Can you work these out from the model? Positions are in its coordinate system, mm. Face numbers are marked on the shaded views. A direction names the side the tool comes from. Coordinates: 2 decimals unless noted, no trailing zeros. Loops run counter-clockwise (first coordinate to the right, second up) from the corner with the lowest first, then second, coordinate; pieces in that order, holes last. Notation, with made-up numbers: M 31,42.5 L 45,42.5 A12 cw 45,60.5 Z; hole C -20.75,20.5 d4. An arc over 180 degrees is marked long. Return JSON: item names as keys, results as strings. Group by question number.
```python
from build123d import *

# Parameters (mm, degrees)
SKETCH1_W                       = 45
SKETCH1_H                       = 20
SKETCH1_R                       = 2.5
BOSS_EXTRUDE1_DEPTH             = 25
SKETCH9_W                       = 45
SKETCH9_H                       = 45
BOSS_EXTRUDE4_DEPTH             = 15
CUT_EXTRUDE2_START              = -2.5
CUT_EXTRUDE2_DEPTH              = 19.5
CHAMFER1_SIZE                   = 10
CBORE_FOR_M5_SBHCS1_D           = 5.5
CBORE_FOR_M5_SBHCS1_CBORE_D     = 10.5
CBORE_FOR_M5_SBHCS1_CBORE_DEPTH = 9.75
CHAMFER2_SIZE                   = 0.5


with BuildPart() as part:
    # Sketch1 → Boss-Extrude1 (new body)
    with BuildSketch(Plane(origin=(0, 0, 0), x_dir=(1, 0, 0), z_dir=(0, 1, 0))):
        Rectangle(SKETCH1_W, SKETCH1_H)
        Circle(SKETCH1_R, mode=Mode.SUBTRACT)
    extrude(amount=BOSS_EXTRUDE1_DEPTH)

    # Sketch9 → Boss-Extrude4 (add)
    with BuildSketch(Plane.XY.offset(10)):
        with Locations((0, 2.5)):
            Rectangle(SKETCH9_W, SKETCH9_H)
    extrude(amount=BOSS_EXTRUDE4_DEPTH)

    # Sketch10 → Cut-Extrude2 (cut)
    with BuildSketch(Plane(origin=(0, 25, 0), x_dir=(1, 0, 0), z_dir=(0, 1, 0)).offset(CUT_EXTRUDE2_START)):
        with BuildLine():
            Line((10.16, 0), (10.16, 10))
            Line((10.16, 10), (-10.16, 10))
            Line((-10.16, 10), (-10.16, 0))
            ThreePointArc((-10.16, 0), (0, -10.16), (10.16, 0))
        make_face()
    extrude(amount=-CUT_EXTRUDE2_DEPTH, mode=Mode.SUBTRACT)

    # Chamfer1
    chamfer1_edges = [part.edges().sort_by_distance(p)[0] for p in [
        (0, 25, 25),
    ]]
    chamfer(chamfer1_edges, length=CHAMFER1_SIZE)

    # CBORE for M5 SBHCS1 (through all)
    with Locations(Plane.XY.offset(25)):
        with Locations((-12.5, -10), (12.5, -10)):
            CounterBoreHole(CBORE_FOR_M5_SBHCS1_D / 2, CBORE_FOR_M5_SBHCS1_CBORE_D / 2, CBORE_FOR_M5_SBHCS1_CBORE_DEPTH)

    # Chamfer2
    chamfer2_edges = [part.edges().sort_by_distance(p)[0] for p in [
        (-22.5, 25, 2.5),
        (-22.5, -20, 17.5),
        (22.5, -20, 17.5),
        (0, -20, 25),
        (22.5, -2.5, 25),
        (-22.5, -2.5, 25),
        (-22.5, 20, 20),
        (22.5, 25, 2.5),
        (22.5, 20, 20),
        (0, 25, -10),
    ]]
    chamfer(chamfer2_edges, length=CHAMFER2_SIZE)


solid = part.part
```
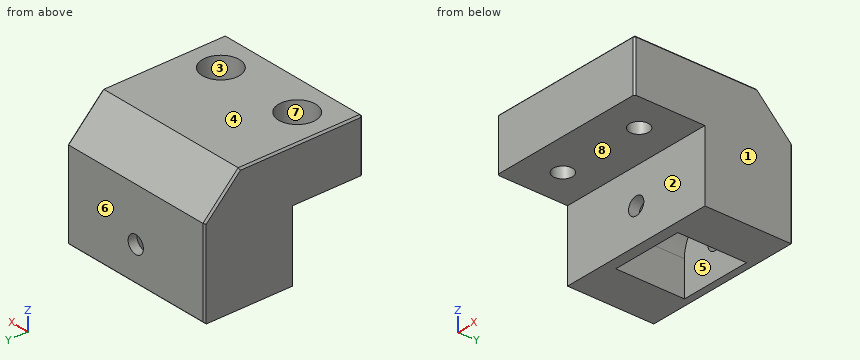
1) Suppose I cut it at B-B, the plane x = 18.5. List the corners of the cut face in (y, z) for me.
2) Suppose I cut it at C-C, the plane z = 22. List the corners of the cut face in (x, y) for me, then the cut area to 3 significant figures.
3) For pin 1 (8.5 mm diameter, centred on x = -12.5, y = -10, fed in from -Z); pin 2 (6.5 mm diameter, centred on x = 12.5, y = -10, fed in from +Z); pin 3 (6 mm diameter, centred on x = 4, z = 4, fed in from -Y), each with a flat end and sliding along its axis, tell me the tip position at first contact or that it passes through.
4) For the marked faces 1, 2, 3, 4 and 5, which set-ups out of +Z, -Z, +X, -X, +Y, -Y let a thin tool reach every point of the face, with its end or its side?
5) If I drill on line 1 (X direction, y = 24, z = 0); line 2 (Y direction, x = 12.5, z = 17.5); line 3 (X direction, y = 9.5, z = -3), over which ranges is the centre line in solid material (lowest first)? Write a range as from..to.
6) If we mould it in two halves opening along Y, with no side actions, what happens to the marked faces 6, 7 and 8? For each: +Y half, -Y half, draft (parallel to the pull), parting line (faces both ways), or undercut.
7) Suppose I cut it at D-D, the plane y = 10. List the corners of the cut face in (x, z) for me, then the cut area to 3 significant figures.
8) Suppose I cut it at A-A, the plane x = -12.5. List the corners of the cut face in (y, z) for me, then the cut area to 4 significant figures.
Returned:
{
 "1": {"outline": "M -20,10 L 0,10 L 0,-10 L 24.5,-10 L 25,-9.5 L 25,15 L 15,25 L -19.5,25 L -20,24.5 Z"},
 "2": {"outline": "M -22.5,-19.5 L -22,-20 L 22,-20 L 22.5,-19.5 L 22.5,17.29 L 22,18 L -22,18 L -22.5,17.29 Z; hole C -12.5,-10 d10.5; hole C 12.5,-10 d10.5", "area": "1,540 mm²"},
 "3": {"pin 1": "stops at z = 10", "pin 2": "stops at z = 15.25", "pin 3": "stops at y = 0"},
 "4": {"face 1": "+Z, -Z, +X, +Y, -Y", "face 2": "-Z, +X, -X, -Y", "face 3": "+Z", "face 4": "+Z, +X, -X, +Y, -Y", "face 5": "-Z"},
 "5": {"line 1": "x = -22.5..-2.5, 2.5..22.5", "line 2": "y = -20..-15.25, -4.75..22.5", "line 3": "x = -22.5..-10.16, 10.16..22.5"},
 "6": {"face 6": "+Y half", "face 7": "undercut", "face 8": "draft"},
 "7": {"outline": "M -22.5,-10 L -10.16,-10 L -10.16,0 A10.16 cw 10.16,0 L 10.16,-10 L 22.5,-10 L 22.5,24.5 L 22,25 L -22,25 L -22.5,24.5 Z", "area": "1,210 mm²"},
 "8": {"outline": "M -20,10 L -12.75,10 L -12.75,15.25 L -15.25,15.25 L -15.25,25 L -19.5,25 L -20,24.5 Z; M -7.25,10 L 0,10 L 0,-10 L 24.5,-10 L 25,-9.5 L 25,15 L 15,25 L -4.75,25 L -4.75,15.25 L -7.25,15.25 Z", "area": "993.5 mm²"}
}
